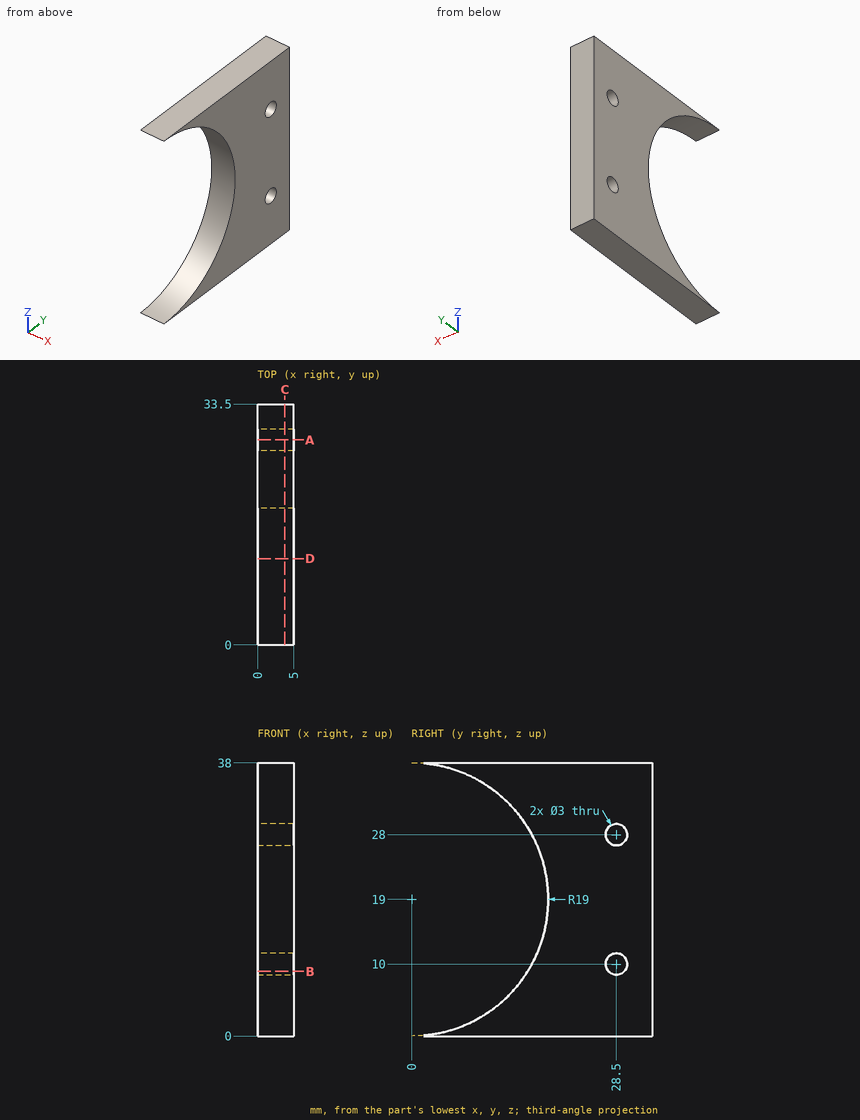
Source: three-view drawing plus pictorial views. Frame: mm from the lowest corner of the part. Coordinates: 2 decimals unless noted, no trailing zeros. Write each loop counter-clockwise with the first axis right and the second up, starting at its lowest first coordinate (ties: lowest second). Pieces come first, ordered by that corner, then holes. Notation, with made-up numbers: (-13, 30.25) -> (42, 30.25) arc R21 ccw to (42, 55.25) -> close; hole circle Ø1 at (57.25, 18). An arc over 180 degrees is marked (long way). Answer as a JSON object with one key per item and string values.
1. Section D-D on y = 12. Return the cut outline in (x, z), then the cut area to 3 significant figures.
Result set:
{"outline": "(0, 0) -> (5, 0) -> (5, 4.27) -> (0, 4.27) -> close; (0, 33.73) -> (5, 33.73) -> (5, 38) -> (0, 38) -> close", "area": "42.7 mm2"}
2. Section B-B on z = 9. Return the cut outline in (x, y).
Result set:
{"outline": "(0, 16.16) -> (5, 16.16) -> (5, 27.38) -> (0, 27.38) -> close; (0, 29.62) -> (5, 29.62) -> (5, 33.5) -> (0, 33.5) -> close"}
3. Material intervals for line 1 (Y direction, x = 2.4, z = 10); line 2 (Y direction, x = 4.35, z = 27); line 3 (Y direction, x = 0.7, z = 19), sorted ascending. Write a range as from..to.
Result set:
{"line 1": "y = 16.73..27, 30..33.5", "line 2": "y = 17.23..27.38, 29.62..33.5", "line 3": "y = 19..33.5"}
4. Section A-A on y = 28.5. Return the cut outline in (x, z), then the cut area to 3 significant figures.
Result set:
{"outline": "(0, 0) -> (5, 0) -> (5, 8.5) -> (0, 8.5) -> close; (0, 11.5) -> (5, 11.5) -> (5, 26.5) -> (0, 26.5) -> close; (0, 29.5) -> (5, 29.5) -> (5, 38) -> (0, 38) -> close", "area": "160 mm2"}
5. Section C-C on x = 3.8. Return the cut outline in (y, z).
Result set:
{"outline": "(0, 0) -> (33.5, 0) -> (33.5, 38) -> (0, 38) arc R19 cw to start; hole circle Ø3 at (28.5, 10); hole circle Ø3 at (28.5, 28)"}
